```python
from build123d import *
from build123d.topology import SkipClean

# Parameters (mm, degrees)
BOSS_EXTRUDE1_DEPTH      = 6.75
BOSS_EXTRUDE1_DEPTH_BACK = 6.75
SKETCH1_R                = 1.7
SKETCH2_R                = 4
BOSS_EXTRUDE2_DEPTH      = 14
SKETCH3_R                = 2.5
CUT_EXTRUDE1_DEPTH       = 5
SKETCH4_R                = 1.7
CUT_EXTRUDE2_DEPTH       = 17.5
CUT_EXTRUDE4_START       = -3
CUT_EXTRUDE4_DEPTH       = 3


with BuildPart() as part:
    # Sketch1 → Boss-Extrude1 (new, two sides: drawn at the far end of the back side and taken through both)
    with BuildSketch(Plane(origin=(0, 0, 0), x_dir=(1, 0, 0), z_dir=(0, 1, 0)).offset(-BOSS_EXTRUDE1_DEPTH_BACK)):
        with BuildLine():
            Line((-3.35, 24), (-3.35, 12))
            ThreePointArc((-3.35, 12), (-4.001241595, 8.033856538), (-5.886575957, 4.484219386))
            ThreePointArc((-5.886575957, 4.484219386), (0, -7.4), (5.886575957, 4.484219386))
            ThreePointArc((5.886575957, 4.484219386), (4.001241595, 8.033856538), (3.35, 12))
            Line((3.35, 12), (3.35, 24))
            ThreePointArc((3.35, 24), (0, 27.35), (-3.35, 24))
        make_face()
        with Locations(Location((0, 24, 0), (0, 0, 270))):
            Circle(SKETCH1_R, mode=Mode.SUBTRACT)
    extrude(amount=BOSS_EXTRUDE1_DEPTH + BOSS_EXTRUDE1_DEPTH_BACK)

    # Sketch2 → Boss-Extrude2 (add)
    with BuildSketch(Plane(origin=(0, 6.75, 0), x_dir=(1, 0, 0), z_dir=(0, 1, 0))):
        with Locations(Location((0, 0, 0), (0, 0, 90))):
            Circle(SKETCH2_R)
    extrude(amount=BOSS_EXTRUDE2_DEPTH)

    # Sketch3 → Cut-Extrude1 (cut)
    with BuildSketch(Plane(origin=(0, 20.75, 0), x_dir=(1, 0, 0), z_dir=(0, 1, 0))):
        with Locations(Location((0, 0, 0), (0, 0, 270))):
            Circle(SKETCH3_R)
    extrude(amount=-CUT_EXTRUDE1_DEPTH, mode=Mode.SUBTRACT)

    # Sketch4 → Cut-Extrude2 (cut)
    with BuildSketch(Plane(origin=(0, 15.75, 0), x_dir=(1, 0, 0), z_dir=(0, 1, 0))):
        with Locations(Location((0, 0, 0), (0, 0, 270))):
            Circle(SKETCH4_R)
    extrude(amount=-CUT_EXTRUDE2_DEPTH, mode=Mode.SUBTRACT)

    # Sketch5 → Cut-Extrude4 (cut)
    with SkipClean():  # the faces are left unmerged after this step: merging them gives an invalid solid
        with BuildSketch(Plane(origin=(0, 6.75, 0), x_dir=(1, 0, 0), z_dir=(0, 1, 0)).offset(CUT_EXTRUDE4_START)):
            with BuildLine():
                Line((3.35, 12), (3.35, 24))
                ThreePointArc((3.35, 24), (0, 27.35), (-3.35, 24))
                Line((-3.35, 24), (-3.35, 12))
                ThreePointArc((-3.35, 12), (-4.001241595, 8.033856538), (-5.886575957, 4.484219386))
                ThreePointArc((-5.886575957, 4.484219386), (0, 7.4), (5.886575957, 4.484219386))
                ThreePointArc((5.886575957, 4.484219386), (4.001241595, 8.033856538), (3.35, 12))
            make_face()
        extrude(amount=CUT_EXTRUDE4_DEPTH, mode=Mode.SUBTRACT)


solid = part.part
```
CAD build for the part. Positions are in the model's coordinates, mm. A direction names the side the tool comes from. Coordinates: 2 decimals unless noted, no trailing zeros. Write each loop counter-clockwise with the first axis right and the second up, starting at its lowest first coordinate (ties: lowest second). Pieces come first, ordered by that corner, then holes.
(1) Two-plate mould, pull along Z, no slides. Class faces 1 (the face through (3.905, 13.652, 0.867)), 2 (the face through (-3.35, -2, -18)), 3 (the face through (-1.66, 7.12, -0.37)): +Z half, -Z half, draft (parallel to the pull), parting line (faces both ways), or undercut.
(2) Cut at A-A, the plane x = 0. List the corners of the cut face in (y, z), and give its area (3 significant figures).
(3) Drill centre lines: probe 1 along X at (y, z) = (-4, -24); probe 2 along X at (y, z) = (12.25, 0); probe 3 along Z at (x, y) = (-1, 3.25). Where is each one in solid material? Low to high.
(4) Cut at D-D, the plane x = -5. List the corners of the cut face in (y, z), and give its area (3 significant figures).
(5) 3-axis set-ups, long thin cutter, end or side, ignore diameter. For faces 4 (the face through (3, 6.75, 3)), 5 (the face through (-0.65, -1.57, -22.43)), 6 (the face through (3.35, -2, -18)): which of +Z, -Z, +X, -X, +Y, -Y reach the whole face in a straight line?
(6) Flat gauge pins, fed straight in: pin 1 (8 mm diameter, centred on x = -1.5, y = 15, fed in from +Z); pin 2 (1.5 mm diameter, centred on x = -5, y = 3.5, fed in from +Z); pin 3 (4 mm diameter, centred on x = 4.5, y = 18, fed in from +Z); pin 4 (2 mm diameter, centred on x = 0, z = -24, fed in from +Y). Where does each tip first touch, or does it go through?
(7) Cut at C-C, the plane y = 10.75. List the corners of the cut face in (x, z).
(8) Cut at B-B, the plane z = 0. List the corners of the cut face in (x, y).
Geometry says:
1. face 1: parting line
1. face 2: draft
1. face 3: undercut
2. outline: (-6.75, -27.35) - (3.75, -27.35) - (3.75, -25.7) - (-6.75, -25.7) - close; (-6.75, -22.3) - (3.75, -22.3) - (3.75, -7.4) - (6.75, -7.4) - (6.75, -4) - (20.75, -4) - (20.75, -2.5) - (15.75, -2.5) - (15.75, -1.7) - (-1.75, -1.7) - (-1.75, 1.7) - (15.75, 1.7) - (15.75, 2.5) - (20.75, 2.5) - (20.75, 4) - (6.75, 4) - (6.75, 7.4) - (-6.75, 7.4) - close
2. area: 401 mm2
3. probe 1: x = -3.35 to -1.7, 1.7 to 3.35
3. probe 2: x = -4 to -1.7, 1.7 to 4
3. probe 3: z = -27.2 to -25.37, -22.63 to -1.37, 1.37 to 7.33
4. outline: (-6.75, -5.82) - (3.75, -5.82) - (3.75, -5.46) - (6.75, -5.46) - (6.75, 5.46) - (-6.75, 5.46) - close
4. area: 151 mm2
5. face 4: +Y
5. face 5: +Y, -Y
5. face 6: -Z, +X, +Y, -Y
6. pin 1: stops at z = 4
6. pin 2: stops at z = 6.06
6. pin 3: stops at z = 3.12
6. pin 4: passes through
7. outline: circle Ø8 at (0, 0); hole circle Ø3.4 at (0, 0)
8. outline: (-7.4, -6.75) - (7.4, -6.75) - (7.4, 6.75) - (4, 6.75) - (4, 20.75) - (2.5, 20.75) - (2.5, 15.75) - (1.7, 15.75) - (1.7, -1.75) - (-1.7, -1.75) - (-1.7, 15.75) - (-2.5, 15.75) - (-2.5, 20.75) - (-4, 20.75) - (-4, 6.75) - (-7.4, 6.75) - close
